```python
from build123d import *

# Parameters (mm, degrees)
F0_R     = 10.125
F1_DEPTH = 15.84
F2_R     = 4
F3_DEPTH = 6.21
F4_R     = 1.3


with BuildPart() as f1:
    # F0 (on Top) → F1 (new body)
    with BuildSketch(Plane.XY):
        with Locations((-14.4086510164, 0)):
            Circle(F0_R)
        with BuildLine():
            ThreePointArc((-9.5045986008, -1.2566527585), (-19.4709204703, -0.0483138353), (-9.529476475, 1.3500229791))
            Line((-9.529476475, 1.3500229791), (-7.7556929707, 1.3500229791))
            Line((-7.7556929707, 1.3500229791), (-7.7556929707, -1.2566527585))
            Line((-7.7556929707, -1.2566527585), (-9.5045986008, -1.2566527585))
        make_face(mode=Mode.SUBTRACT)
    extrude(amount=F1_DEPTH)

    # F2 (on face) → F3 (join)
    with BuildSketch(Plane.XY.offset(15.84)):
        with BuildLine():
            ThreePointArc((4.2266686103, -7.4980342454), (9.4186281084, -5.2422426418), (11.5549640544, 0))
            ThreePointArc((11.5549640544, 0), (9.500818026, 5.1568085595), (4.4635841825, 7.4888603666))
            ThreePointArc((4.4635841825, 7.4888603666), (-3.4440990013, 0.1185465609), (4.2266686103, -7.4980342454))
        make_face()
        with Locations((4.0549640544, 0)):
            Circle(F2_R, mode=Mode.SUBTRACT)
        with BuildLine():
            ThreePointArc((4.2266686103, -7.4980342454), (-3.4440990013, 0.1185465609), (4.4635841825, 7.4888603666))
            Line((4.4635841825, 7.4888603666), (-11.8889977578, 9.8064760468))
            ThreePointArc((-11.8889977578, 9.8064760468), (-6.4078037412, 6.2050034551), (-4.2836510164, 0))
            ThreePointArc((-4.2836510164, 0), (-6.3377093937, -6.113552676), (-11.6664710308, -9.7465929394))
            Line((-11.6664710308, -9.7465929394), (4.2266686103, -7.4980342454))
        make_face()
    extrude(amount=-F3_DEPTH)

    # F4
    f4_edges = [f1.edges().sort_by_distance(p)[0] for p in [
        (-24.533651, 0, 0),
    ]]
    fillet(f4_edges, radius=F4_R)


solid = f1.part
```
The model under review builds one solid part; all positions refer to its coordinate system, in mm. A direction names the side the tool comes from. Round coordinates to 2 decimals unless told otherwise and drop trailing zeros. Loops run counter-clockwise (first coordinate to the right, second up) from the corner with the lowest first, then second, coordinate; pieces in that order, holes last.
Item 1: Mouldability with a two-part tool opening along X and no side actions: class faces 1 (the face through (-7, 0, 15.84)), 2 (the face through (-3.831, -8.638, 12.778)), 3 (the face through (-19.465, -0.252, 7.809)) as released by +X, released by -X, zero draft, split by the parting line, or undercut.
Determined:
face 1: zero draft
face 2: released by +X
face 3: undercut
Item 2: For line 1 (X direction, y = -0.25, z = 1.25); line 2 (Z direction, x = 0, y = 3.5); line 3 (X direction, y = -0.5, z = 11.5), list the stretches that pass through material, from the lowest coordinate up.
Determined:
line 1: x = -24.53 to -19.46, -7.76 to -4.29
line 2: z = 9.63 to 15.84
line 3: x = -24.52 to -19.45, -7.76 to 0.09, 8.02 to 11.54
Item 3: Take a section at A-A (x = 6). Write out the cut boundary in (y, z), then the cut area to 3 significant figures.
Determined:
outline: (-7.24, 9.63) - (-3.5, 9.63) - (-3.5, 15.84) - (-7.24, 15.84) - close; (3.5, 9.63) - (7.24, 9.63) - (7.24, 15.84) - (3.5, 15.84) - close
area: 46.6 mm2
Item 4: Clearance check with flat-ended pins moving along their axes: pin 1 Ø4 at (y, z) = (1, 8.5) entering from +X; pin 2 Ø6 at (y, z) = (-7, 6.5) entering from +X; pin 3 Ø1 at (x, z) = (-9, 8) entering from +Y; pin 4 Ø0.9 at (x, z) = (-8.5, 10.5) entering from -Y. State where each tip first meets the part, or that it passes through.
Determined:
pin 1: stops at x = 11.55
pin 2: stops at x = -5.11
pin 3: stops at y = 8.86
pin 4: stops at y = -9.36
Item 5: For faces 4 (the face through (-11, -4, 0)), 5 (the face through (-7.756, 0, 8)), 6 (the face through (-24.524, 0.445, 6.853)), list the 3-axis set-ups (+Z, -Z, +X, -X, +Y, -Y) from which the entire face can be reached by the end or side of a thin tool; tool diameter is ignored.
Determined:
face 4: -Z, +X, -X, +Y, -Y
face 5: +Z, -Z
face 6: -Z
Item 6: Take a section at C-C (z = 14.75). Give the number of separate pieces and of enclosed holes in the cut face, then the cut area to 3 significant figures.
Determined:
separate pieces: 1
enclosed holes: 2
area: 441 mm2
